The model under review builds one solid part; all positions refer to its coordinate system, in mm. Round coordinates to 2 decimals unless told otherwise and drop trailing zeros. Write each loop counter-clockwise with the first axis right and the second up, starting at its lowest first coordinate (ties: lowest second). Pieces come first, ordered by that corner, then holes. Notation, with made-up numbers: (-2.5, 5) - (52.5, 5) arc R22 ccw to (52.5, 26) - close; hole circle Ø4 at (46, 30.25). An arc over 180 degrees is marked (long way). Use one line per item in the form item = value.
Autodesk Inventor part; units mm, degrees
ref_plane "YZ Plane" through (0, 0, 0) normal (1, 0, 0) x (0, 1, 0)
ref_plane "XZ Plane" through (0, 0, 0) normal (0, 1, 0) x (-1, 0, 0)
ref_plane "XY Plane" through (0, 0, 0) normal (0, 0, 1) x (1, 0, 0)
sketch "Sketch1" plane through (0, 0, 0) normal (0, 1, 0) x (-1, 0, 0)
  line L0 (0, 0) -> (0, -9.525)
  arc A0 (6.35, 0) -> (-6.35, 0) centre (0, 0) ccw
  line L1 (6.35, 0) -> (6.35, -9.525)
  line L2 (-6.35, 0) -> (-6.35, -9.525)
  line L3 (6.35, -9.525) -> (0, -33.2235)
  line L4 (0, -33.2235) -> (-6.35, -9.525)
  dimension "d0" = 9.525
  dimension "d1" = 12.7
  dimension "d13" = 165
  dimension "d14" = 9.525
  dimension "d15" = 9.525
  dimension "d16" = 165
extrude "Extrusion1" add sketch "Sketch1" along normal blind 3.175
hole "Hole1" at (0, 0, 0) at (0, 0, -9.525) direction (0, 1, 0) diameter 4.9784 end through all
equation "\"d1\" = thickness"
equation "\"height\" = 203.2"
equation "\"thickness\" = 12.7"
equation "\"shaftDiam\" = 6.35"
equation "\"shaftSpace\" = 1.5875"
equation "\"stageSpace\" = 2.54"
equation "\"stageAngle\" = 15deg"
equation "\"bearingDiam\" = 9.5504"
equation "\"FlangeDiam\" = 12.7"
equation "\"FlangeDepth\" = 1.5875"
equation "\"smallFilet\" = 0.39687"
equation "\"ringDiam\" = 96.46608"
equation "\"stockHeight\" = 50.8"
equation "\"stockWidth\" = 76.2"
equation "\"stockRad\" = 9.525"
equation "\"stockGuage\" = 3.175"
equation "\"groundActu\" = 304.8"
equation "\"baseWidth\" = 1066.8"
equation "\"baseDepth\" = 254"
equation "\"capThickness\" = 3.175"
equation "\"sup1Len\" = 660.4"
equation "\"sup1Ang\" = 22.619865deg"
equation "\"sup2Len\" = 2079.37366"
equation "\"sup2Ang\" = 8.959949deg"
equation "\"supVertLen\" = 955.13561"
equation "\"supSideLen\" = 1531.12879"
equation "\"supSideAng\" = 19.376933deg"
properties part number "lock ring 2 supp" material "Aluminum 6061"
(1) Add section D-D on x = -0.75. Write out the cut boundary in (y, z) (3 decimals).
Geometry results:
outline = (0, -30.424) - (3.175, -30.424) - (3.175, -11.899) - (0, -11.899) - close; (0, -7.151) - (3.175, -7.151) - (3.175, -2.374) - (0, -2.374) - close; (0, 2.374) - (3.175, 2.374) - (3.175, 6.306) - (0, 6.306) - close
(2) Add section B-B on x = 1.5. Write out the cut boundary in (y, z) (3 decimals).
Geometry results:
outline = (0, -27.625) - (3.175, -27.625) - (3.175, -11.511) - (0, -11.511) - close; (0, -7.539) - (3.175, -7.539) - (3.175, -1.986) - (0, -1.986) - close; (0, 1.986) - (3.175, 1.986) - (3.175, 6.17) - (0, 6.17) - close
(3) Insertion check: P1, Ø1, axis at y = 3, z = -25, coming from the +X side. The pin has a flat end and moves straight along its axis. Give the tip position at first contact, or say it passes through.
Geometry results:
P1 = 2.34
(4) The part is to be moulded in two halves that separate along X. For faces 1 (the cylindrical face through (-0.748, 1.61, -2.374)), 2 (the flat face through (-3, 3.175, -9)), 3 (the flat face through (-3.22, 1.57, -21.21)), say which applies: +X half, -X half, draft (parallel to the pull), parting line (faces both ways), or undercut.
Geometry results:
face_1 = undercut
face_2 = draft
face_3 = -X half
(5) Add section A-A on y = 0.7. Count the separate pieces of the cut face and the enclosed holes in it, then the cut area to 3 significant figures.
Geometry results:
separate_pieces = 1
enclosed_holes = 2
area = 296 mm2
(6) Add section C-C on z = 1. Write out the cut boundary in (x, y) (1 decimal).
Geometry results:
outline = (-6.3, 0) - (-2.3, 0) - (-2.3, 3.2) - (-6.3, 3.2) - close; (2.3, 0) - (6.3, 0) - (6.3, 3.2) - (2.3, 3.2) - close
(7) To check wall thickness, follow L1, parallel to X at y = 0.95, z = 0; L2, parallel to X at y = 1.2, z = 0.5; L3, parallel to X at y = 1.5, z = -25. State the ranges of each line that lie inside material, in increasing order.
Geometry results:
L1 = -6.35 to -2.49, 2.49 to 6.35
L2 = -6.33 to -2.44, 2.44 to 6.33
L3 = -2.2 to 2.2
